Verification items for this drawing (mm, ordinates from the low corner). Round coordinates to 2 decimals unless told otherwise and drop trailing zeros. Write each loop counter-clockwise with the first axis right and the second up, starting at its lowest first coordinate (ties: lowest second). Pieces come first, ordered by that corner, then holes.
Item 1: Cross-section at B-B (z = 6.35). Enter the section's corners in (x, y) (1 decimal).
Item 2: Draft check along Z on the marked faces 1, 2, 3 and 4. Enter one of: pulls with the +Z half, pulls with the -Z half, needs draft (parallel to the pull), parting line crosses it, or undercut.
Item 3: Cross-section at C-C (y = 6). Enter the section's corners in (x, z).
Item 4: Depth check by flat-ended pin: P1, Ø2.5, axis at x = 42.98, z = 19.05, coming from the -Y side. Enter the tip coordinate at first touch or a pass-through.
Item 5: Scan lines: probe 1 along Z at (x, y) = (43, 2.75); probe 2 along X at (y, z) = (16.5, 19.5) (1 decimal); probe 3 along Z at (x, y) = (42, 4.25) (1 decimal). Record each from-to range of solid material in increasing order.
Item 6: Cross-section at A-A (x = 6.35). Enter the section's corners in (y, z), then the cut area to 3 significant figures.
Item 7: Cross-section at D-D (y = 14.75). Enter the section's corners in (x, z).
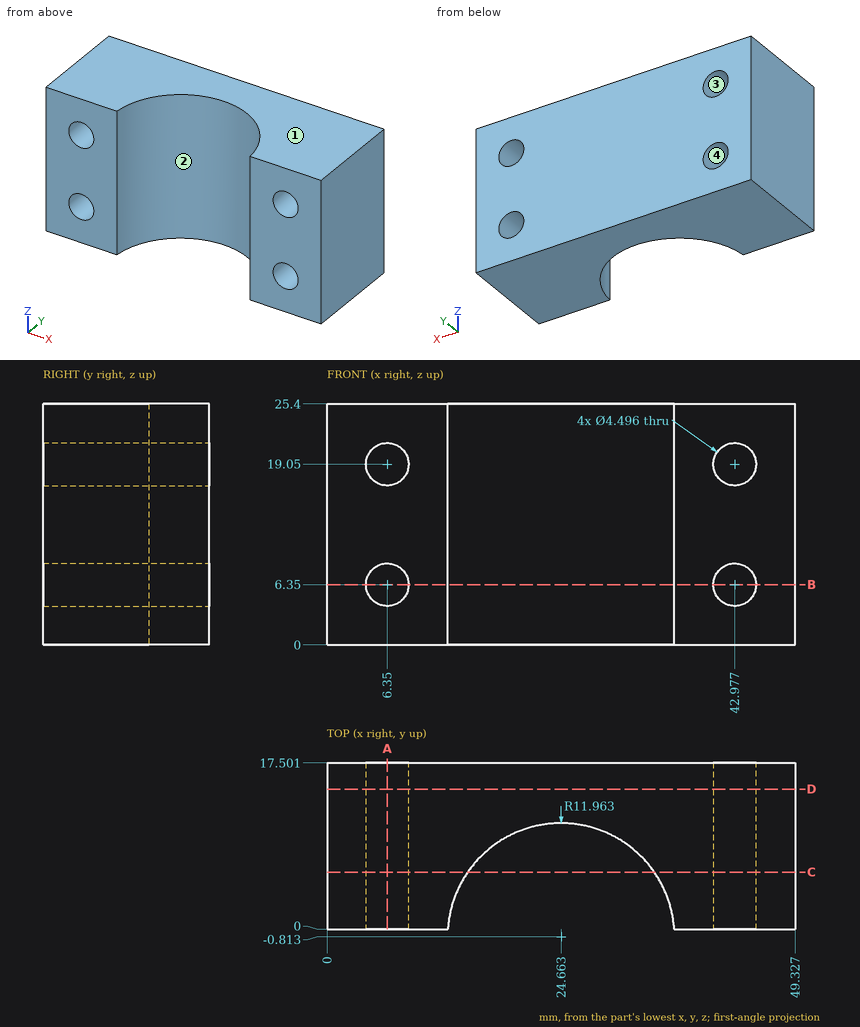
Resolved:
1. outline: (0, 0) - (4.1, 0) - (4.1, 17.5) - (0, 17.5) - close; (8.6, 0) - (12.7, 0) arc R12 cw to (36.6, 0) - (40.7, 0) - (40.7, 17.5) - (8.6, 17.5) - close; (45.2, 0) - (49.3, 0) - (49.3, 17.5) - (45.2, 17.5) - close
2. face 1: pulls with the +Z half
2. face 2: needs draft
2. face 3: undercut
2. face 4: undercut
3. outline: (0, 0) - (14.83, 0) - (14.83, 25.4) - (0, 25.4) - close; (34.5, 0) - (49.33, 0) - (49.33, 25.4) - (34.5, 25.4) - close; hole circle Ø4.5 at (6.35, 6.35); hole circle Ø4.5 at (6.35, 19.05); hole circle Ø4.5 at (42.98, 6.35); hole circle Ø4.5 at (42.98, 19.05)
4. P1: passes through
5. probe 1: z = 0 to 4.1, 8.6 to 16.8, 21.3 to 25.4
5. probe 2: x = 0 to 4.1, 8.6 to 40.8, 45.2 to 49.3
5. probe 3: z = 0 to 4.3, 8.4 to 17, 21.1 to 25.4
6. outline: (0, 0) - (17.5, 0) - (17.5, 4.1) - (0, 4.1) - close; (0, 8.6) - (17.5, 8.6) - (17.5, 16.8) - (0, 16.8) - close; (0, 21.3) - (17.5, 21.3) - (17.5, 25.4) - (0, 25.4) - close
6. area: 287 mm2
7. outline: (0, 0) - (49.33, 0) - (49.33, 25.4) - (0, 25.4) - close; hole circle Ø4.5 at (6.35, 6.35); hole circle Ø4.5 at (6.35, 19.05); hole circle Ø4.5 at (42.98, 6.35); hole circle Ø4.5 at (42.98, 19.05)
